from build123d import *

# Parameters (mm, degrees)
SKETCH1_R               = 69.05625
BOSS_EXTRUDE1_DEPTH     = 6.35
F_1_4_CLEARANCE_HOLE1_D = 7.14248
F_3_8_CLEARANCE_HOLE1_D = 10.31748
SKETCH6_R               = 3.57124
CUT_EXTRUDE1_DEPTH      = 6.35


with BuildPart() as part:
    # Sketch1 → Boss-Extrude1 (new body)
    with BuildSketch(Plane(origin=(0, 0, 0), x_dir=(1, 0, 0), z_dir=(0, 1, 0))):
        Circle(SKETCH1_R)
    extrude(amount=BOSS_EXTRUDE1_DEPTH)

    # 1/4 Clearance Hole1 (through all)
    with Locations(Plane(origin=(0, 6.35, 0), x_dir=(1, 0, 0), z_dir=(0, 1, 0))):
        with Locations((0, 0)):
            Hole(F_1_4_CLEARANCE_HOLE1_D / 2)

    # 3/8 Clearance Hole1 (through all)
    with Locations(Plane(origin=(0, 6.35, 0), x_dir=(1, 0, 0), z_dir=(0, 1, 0))):
        with Locations((0, 26.9875), (0, -26.9875)):
            Hole(F_3_8_CLEARANCE_HOLE1_D / 2)

    # Sketch6 → Cut-Extrude1 (cut)
    with BuildSketch(Plane(origin=(0, 6.35, 0), x_dir=(1, 0, 0), z_dir=(0, 1, 0))):
        with Locations((15.1384, -15.5575)):
            Circle(SKETCH6_R)
    extrude(amount=-CUT_EXTRUDE1_DEPTH, mode=Mode.SUBTRACT)


solid = part.part
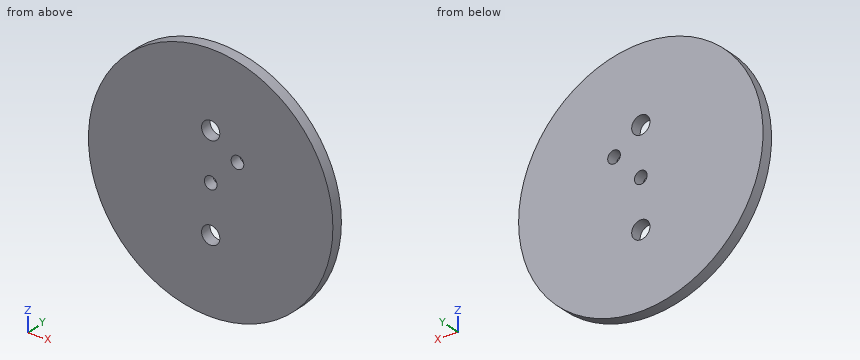
Work out the finished part from the listing and answer in its coordinate system (mm). Coordinates: 2 decimals unless noted, no trailing zeros. Write each loop counter-clockwise with the first axis right and the second up, starting at its lowest first coordinate (ties: lowest second). Pieces come first, ordered by that corner, then holes. Notation, with made-up numbers: M 45.25,-30 L 98.25,-30 A21 cw 98.25,-4 Z; hole C 25,73 d8. An arc over 180 degrees is marked long. Write item = value, one per line.
1. The part is cut by section C-C (y = 1). Determine the outline of the cut face in (x, z), then the cut area to 3 significant figures.
Solution:
outline = C 0,0 d138.11; hole C 0,-26.99 d10.32; hole C 0,26.99 d10.32; hole C 0,0 d7.14; hole C 15.14,15.56 d7.14
area = 14,700 mm2
2. The part is cut by section B-B (z = 0). Determine the outline of the cut face in (x, y).
Solution:
outline = M -69.06,0 L -3.57,0 L -3.57,6.35 L -69.06,6.35 Z; M 3.57,0 L 69.06,0 L 69.06,6.35 L 3.57,6.35 Z
3. Flat-ended cylindrical pins translate along their axes: pin 1 (4 mm diameter, centred on x = -31, z = -46, fed in from -Y); pin 2 (1 mm diameter, centred on x = 51, y = 4, fed in from -Z); pin 3 (1 mm diameter, centred on x = -27.5, y = 1, fed in from -Z). Find the tip coordinate at first contact, or state that the pin passes through.
Solution:
pin_1 = 0
pin_2 = -47.1
pin_3 = -63.56
4. The part is cut by section A-A (x = 0). Determine the outline of the cut face in (y, z), then the cut area to 3 significant figures.
Solution:
outline = M 0,-69.06 L 6.35,-69.06 L 6.35,-32.15 L 0,-32.15 Z; M 0,-21.83 L 6.35,-21.83 L 6.35,-3.57 L 0,-3.57 Z; M 0,3.57 L 6.35,3.57 L 6.35,21.83 L 0,21.83 Z; M 0,32.15 L 6.35,32.15 L 6.35,69.06 L 0,69.06 Z
area = 701 mm2
5. The part is cut by section D-D (z = 30). Determine the outline of the cut face in (x, y).
Solution:
outline = M -62.2,0 L -4.19,0 L -4.19,6.35 L -62.2,6.35 Z; M 4.19,0 L 62.2,0 L 62.2,6.35 L 4.19,6.35 Z
6. Straight lines are drawn through the part: line 1 (Z direction, x = 0, y = 3.25); line 2 (X direction, y = 3.75, z = 38); line 3 (X direction, y = 2, z = -11). For each, find the intervals that lie inside material, in ascending order. Write a range as from..to.
Solution:
line_1 = -69.06..-32.15, -21.83..-3.57, 3.57..21.83, 32.15..69.06
line_2 = -57.66..57.66
line_3 = -68.17..68.17
